Input: part model. Units: mm. Frame: model coordinates. A direction names the side the tool comes from. Give positions to 0.01 mm unless a question says otherwise; leave off trailing zeros. Loops run counter-clockwise (first coordinate to the right, second up) from the corner with the lowest first, then second, coordinate; pieces in that order, holes last. Notation, with made-up numbers: M 18.5,66.25 L 55.5,66.25 A20 ccw 55.5,96.25 Z; hole C -4.75,42.5 d7. An arc over 180 degrees is marked long. Use CSV: the item, a comma, the result in double quotes. Start each with the question number.
Q1. Section A-A, the plane x = 3.5. Output: boundary loops of the cut face in (y, z).
Q2. Material intervals for line 1 along X through (y, z) = (3.5, -7.5); line 2 along Y through (x, z) = (23, -9.5), sorted ascending.
Q3. Reachability of faces 4 (the flat face through (13.3, 27, 0.3)), 5 (the cylindrical face through (28.715, 4.699, -4.127)), 6 (the cylindrical face through (4.715, 22.301, -8.907)), 7 (the flat face through (13.4, 27.5, 0)), 8 (the cylindrical face through (13.633, -1.699, 0.285)) from +Z, -Z, +X, -X, +Y, -Y: full face, straight path, thin tool, end or side. Return the list, or none.
Q4. Section C-C, the plane z = 0.5. Output: boundary loops of the cut face in (x, y).
Q5. Section D-D, the plane x = 21. Output: boundary loops of the cut face in (y, z).
Q6. Pull-direction query (X, two-part tool) for faces 1 (the flat face through (3, 3, -8.4)), 2 (the cylindrical face through (-1.715, 22.301, -4.127)), 3 (the flat face through (2, 2, -10.4)); classes: released by +X, released by -X, zero draft, split by the parting line, or undercut.
Q7. Pin query (flat end, axial travel): pin 1 (1.1 mm diameter, centred on x = 16, y = 27.5, fed in from -Z); pin 2 (1 mm diameter, centred on x = 21, z = -5.5, fed in from -Y); pin 3 (1.5 mm diameter, centred on x = 1.5, y = 24.5, fed in from +Z); pin 4 (4 mm diameter, centred on y = 20.5, z = -3.5, fed in from +X). Return the tip coordinate at first contact, or that it passes through.
from build123d import *

# Parameters (mm, degrees)
SKETCH1_W           = 31
SKETCH1_H           = 31
SKETCH1_W_2         = 27
SKETCH1_H_2         = 27
BOSS_EXTRUDE1_DEPTH = 2
BOSS_EXTRUDE2_DEPTH = 8.4
SKETCH4_W           = 7
SKETCH4_H           = 7
BOSS_EXTRUDE3_DEPTH = 2
FILLET1_R           = 1


with BuildPart() as part:
    # Sketch1 → Boss-Extrude1 (new body)
    with BuildSketch(Plane.XY):
        with Locations((13.5, 13.5)):
            Rectangle(SKETCH1_W, SKETCH1_H)
        with Locations((13.5, 13.5)):
            Rectangle(SKETCH1_W_2, SKETCH1_H_2, mode=Mode.SUBTRACT)
    extrude(amount=BOSS_EXTRUDE1_DEPTH)

    # Sketch2 → Boss-Extrude2 (add)
    with BuildSketch(Plane(origin=(0, 0, 0), x_dir=(-1, 0, 0), z_dir=(0, 0, -1))):
        Polygon((-29, 29), (-22, 29), (-22, 27), (-27, 27), (-27, 22), (-29, 22), align=None)
        Polygon((2, 29), (-5, 29), (-5, 27), (0, 27), (0, 22), (2, 22), align=None)
        Polygon((2, 5), (2, -2), (-5, -2), (-5, 0), (0, 0), (0, 5), align=None)
        Polygon((-29, -2), (-29, 5), (-27, 5), (-27, 0), (-22, 0), (-22, -2), align=None)
    extrude(amount=BOSS_EXTRUDE2_DEPTH)

    # Sketch4 → Boss-Extrude3 (add)
    with BuildSketch(Plane(origin=(0, 0, -8.4), x_dir=(-1, 0, 0), z_dir=(0, 0, -1))):
        with Locations((-25.5, 25.5)):
            Rectangle(SKETCH4_W, SKETCH4_H)
        with Locations((-25.5, 1.5)):
            Rectangle(SKETCH4_W, SKETCH4_H)
        with Locations((-1.5, 1.5)):
            Rectangle(SKETCH4_W, SKETCH4_H)
        with Locations((-1.5, 25.5)):
            Rectangle(SKETCH4_W, SKETCH4_H)
    extrude(amount=BOSS_EXTRUDE3_DEPTH)

    # Fillet1
    fillet1_edges = [part.edges().sort_by_distance(p)[0] for p in [
        (-2, 25.5, -10.4),
        (1.5, 29, -10.4),
        (-2, 29, -4.2),
        (-2, 22, -5.2),
        (5, 5, -9.4),
        (-2, 5, -5.2),
        (-2, 13.5, 0),
        (-2, -2, -4.2),
        (5, 1.5, -10.4),
        (1.5, 5, -10.4),
        (-2, 1.5, -10.4),
        (1.5, -2, -10.4),
        (5, -2, -5.2),
        (13.5, -2, 0),
        (22, 5, -9.4),
        (22, -2, -5.2),
        (29, -2, -4.2),
        (25.5, -2, -10.4),
        (22, 22, -9.4),
        (5, 22, -9.4),
        (22, 1.5, -10.4),
        (25.5, 5, -10.4),
        (29, 1.5, -10.4),
        (29, 5, -5.2),
        (29, 13.5, 0),
        (29, 29, -4.2),
        (29, 22, -5.2),
        (29, 25.5, -10.4),
        (25.5, 22, -10.4),
        (25.5, 29, -10.4),
        (22, 25.5, -10.4),
        (22, 29, -5.2),
        (13.5, 29, 0),
        (5, 29, -5.2),
        (1.5, 22, -10.4),
        (5, 25.5, -10.4),
    ]]
    fillet(fillet1_edges, radius=FILLET1_R)


solid = part.part
A:
1,outline,"M -2,-9.4 A1 ccw -1,-10.4 L 4,-10.4 A1 ccw 5,-9.4 L 5,-8.4 L 0,-8.4 L 0,2 L -2,2 Z; M 22,-9.4 A1 ccw 23,-10.4 L 28,-10.4 A1 ccw 29,-9.4 L 29,2 L 27,2 L 27,-8.4 L 22,-8.4 Z"
2,line 1,"-2 to 0, 27 to 29"
2,line 2,"-1.99 to 4.99, 22.01 to 28.99"
3,face 4,"+Z"
3,face 5,"-Z, +X"
3,face 6,"+Z, -Z"
3,face 7,"-Z, +Y, -Y"
3,face 8,"-Z, -Y"
4,outline,"M -2,-1 A1 ccw -1,-2 L 4,-2 A1 ccw 4.5,-1.87 L 22.5,-1.87 A1 ccw 23,-2 L 28,-2 A1 ccw 29,-1 L 29,4 A1 ccw 28.87,4.5 L 28.87,22.5 A1 ccw 29,23 L 29,28 A1 ccw 28,29 L 23,29 A1 ccw 22.5,28.87 L 4.5,28.87 A1 ccw 4,29 L -1,29 A1 ccw -2,28 L -2,23 A1 ccw -1.87,22.5 L -1.87,4.5 A1 ccw -2,4 Z; hole M 0,0 L 27,0 L 27,27 L 0,27 Z"
5,outline,"M -2,1 A1 ccw -1,0 L 0,0 L 0,2 L -2,2 Z; M 27,0 L 28,0 A1 ccw 29,1 L 29,2 L 27,2 Z"
6,face 1,"undercut"
6,face 2,"released by -X"
6,face 3,"zero draft"
7,pin 1,"z = 0"
7,pin 2,"through"
7,pin 3,"z = -8.4"
7,pin 4,"x = 28.87"
